from build123d import *

# Parameters (mm, degrees)
SKETCH1_R             = 75
SKETCH1_R_2           = 38
BOSS_EXTRUDE1_DEPTH   = 38
BOSS_EXTRUDE1_2_DEPTH = 38
BOSS_EXTRUDE2_DEPTH   = 23.574371523


with BuildPart() as part:
    # Sketch1 → Boss-Extrude1 (new, symmetric)
    with BuildSketch(Plane.XY):
        Circle(SKETCH1_R)
        Circle(SKETCH1_R_2, mode=Mode.SUBTRACT)
    extrude(amount=BOSS_EXTRUDE1_DEPTH, both=True)



with BuildPart() as body_2:
    # Sketch1 → Boss-Extrude1 2 (new, symmetric)
    with BuildSketch(Plane.XY):
        with Locations((610, 0)):
            Circle(SKETCH1_R)
        with Locations((610, 0)):
            Circle(SKETCH1_R_2, mode=Mode.SUBTRACT)
    extrude(amount=BOSS_EXTRUDE1_2_DEPTH, both=True)


with BuildPart() as part_1:
    add(part.part)

    add(body_2.part)  # Boss-Extrude2 merges body 2
    # Sketch2 → Boss-Extrude2 (add, symmetric)
    with BuildSketch(Plane.XY):
        with BuildLine():
            ThreePointArc((75, 0), (71.203239503, -23.560532341), (60.197368421, -44.735632724))
            ThreePointArc((60.197368421, -44.735632724), (305, 78.339460867), (549.802631579, -44.735632724))
            ThreePointArc((549.802631579, -44.735632724), (566.27585101, 60.936022147), (671.657681941, 42.700471399))
            ThreePointArc((671.657681941, 42.700471399), (305, 234.775001479), (-61.657681941, 42.700471399))
            ThreePointArc((-61.657681941, 42.700471399), (22.368212428, 71.586752076), (75, 0))
        make_face()
    extrude(amount=BOSS_EXTRUDE2_DEPTH, both=True)


solid = part_1.part
The model under review builds one solid part; all positions refer to its coordinate system, in mm. A direction names the side the tool comes from. Coordinates: 2 decimals unless noted, no trailing zeros. Write each loop counter-clockwise with the first axis right and the second up, starting at its lowest first coordinate (ties: lowest second). Pieces come first, ordered by that corner, then holes. Notation, with made-up numbers: (-28.5, 58.5) - (7.5, 58.5) arc R18 cw to (7.5, 77.5) - close; hole circle Ø8 at (40, -24). An arc over 180 degrees is marked (long way). Answer as CSV lines item,"result".
(1) We need section A-A (z = 12). Give the boundary of the cut face in (x, y) (3 decimals).
Data:
outline,"(-61.658, 42.7) arc R75 ccw to (60.197, -44.736) arc R305 cw to (549.803, -44.736) arc R75 ccw to (671.658, 42.7) arc R446 ccw to start; hole circle Ø76 at (0, 0); hole circle Ø76 at (610, 0)"
(2) We need section D-D (x = 610). Give the boundary of the cut face in (y, z).
Data:
outline,"(-75, -38) - (-38, -38) - (-38, 38) - (-75, 38) - close; (38, -38) - (75, -38) - (75, -23.57) - (114.18, -23.57) - (114.18, 23.57) - (75, 23.57) - (75, 38) - (38, 38) - close"
(3) Mouldability with a two-part tool opening along Y and no side actions: class faces 3 (the cylindrical face through (-16.259, -73.217, 0.532)), 4 (the cylindrical face through (17.535, -33.713, -0.532)), 5 (the flat face through (576, 18, 38)) as pulls with the +Y half, pulls with the -Y half, needs draft (parallel to the pull), parting line crosses it, or undercut.
Data:
face 3,"parting line crosses it"
face 4,"undercut"
face 5,"needs draft"
(4) For line 1 along X through (y, z) = (3, 17); line 2 along X through (y, z) = (30.5, 11.5); line 3 along Z through (x, y) = (342, 114.5), list the stretches that pass through material, from the lowest coordinate up. Write a range as [from, to].
Data:
line 1,"x = [-74.94, -37.88], [37.88, 104.3], [505.7, 572.12], [647.88, 684.94]"
line 2,"x = [-68.52, -22.67], [22.67, 141.01], [468.99, 587.33], [632.67, 678.52]"
line 3,"z = [-23.57, 23.57]"
(5) Tool access review of faces 1 (the flat face through (576, 18, -38)), 2 (the cylindrical face through (644.608, -66.538, 0.532)): name each direction out of +Z, -Z, +X, -X, +Y, -Y from which nothing blocks a thin tool from reaching the whole face with its end or side.
Data:
face 1,"-Z, +X, -X, +Y, -Y"
face 2,"none"
(6) Clearance check with flat-ended pins moving along their axes: pin 1 Ø8 at (x, y) = (82, 92.5) entering from +Z; pin 2 Ø6 at (y, z) = (180.5, 20) entering from +X; pin 3 Ø4 at (x, z) = (10.5, 1) entering from -Y. State where each tip first meets the part, or that it passes through.
Data:
pin 1,"stops at z = 23.57"
pin 2,"stops at x = 523.65"
pin 3,"stops at y = -74.52"
(7) We need section B-B (x = -14). Give the boundary of the cut face in (y, z), plus the area to 3 significant figures.
Data:
outline,"(-73.68, -38) - (-35.33, -38) - (-35.33, 38) - (-73.68, 38) - close; (35.33, -38) - (73.68, -38) - (73.68, -23.57) - (100.47, -23.57) - (100.47, 23.57) - (73.68, 23.57) - (73.68, 38) - (35.33, 38) - close"
area,"7,090 mm2"
(8) We need section C-C (y = 0). Give the boundary of the cut face in (x, z).
Data:
outline,"(-75, -38) - (-38, -38) - (-38, 38) - (-75, 38) - close; (38, -38) - (75, -38) - (75, -23.57) - (100.92, -23.57) - (100.92, 23.57) - (75, 23.57) - (75, 38) - (38, 38) - close; (509.08, -23.57) - (535, -23.57) - (535, -38) - (572, -38) - (572, 38) - (535, 38) - (535, 23.57) - (509.08, 23.57) - close; (648, -38) - (685, -38) - (685, 38) - (648, 38) - close"
